```python
from build123d import *

# Parameters (mm, degrees)
SKETCH1_W           = 95.25
SKETCH1_H           = 127
BOSS_EXTRUDE1_DEPTH = 6.35
BOSS_EXTRUDE3_DEPTH = 6.35
SKETCH5_R           = 4.826
CUT_EXTRUDE1_DEPTH  = 7.35
CUT_EXTRUDE2_DEPTH  = 7.35
FILLET9_R           = 5
SKETCH7_R           = 5.453804141
BOSS_EXTRUDE4_DEPTH = 6.35
SKETCH8_W           = 69.85
SKETCH8_H           = 101.6
CUT_EXTRUDE3_DEPTH  = 3.175
SKETCH9_W           = 57.15
SKETCH9_H           = 88.9
CUT_EXTRUDE4_DEPTH  = 4.175
SKETCH11_R          = 1.5875
CUT_EXTRUDE6_DEPTH  = 4.175
CUT_EXTRUDE7_DEPTH  = 3.175
FILLET10_R          = 5
FILLET11_R          = 5
FILLET12_R          = 7.62
SKETCH13_R          = 2.2812375
CUT_EXTRUDE8_DEPTH  = 7.35


with BuildPart() as part:
    # Sketch1 → Boss-Extrude1 (new body)
    with BuildSketch(Plane(origin=(0, 0, 0), x_dir=(1, 0, 0), z_dir=(0, 1, 0))):
        Rectangle(SKETCH1_W, SKETCH1_H)
    extrude(amount=BOSS_EXTRUDE1_DEPTH)

    # Sketch4 → Boss-Extrude3 (add)
    with BuildSketch(Plane(origin=(0, 6.35, 0), x_dir=(1, 0, 0), z_dir=(0, 1, 0))):
        with BuildLine():
            Line((-47.625, 63.5), (-171.916018217, 24.219268021))
            ThreePointArc((-171.916018217, 24.219268021), (-189.6618, 0), (-171.916018217, -24.219268021))
            Line((-171.916018217, -24.219268021), (-47.625, -63.5))
            Line((-47.625, -63.5), (-47.625, 63.5))
        make_face()
    extrude(amount=-BOSS_EXTRUDE3_DEPTH)

    # Sketch5 → Cut-Extrude1 (cut, through all)
    with BuildSketch(Plane(origin=(0, 6.35, 0), x_dir=(1, 0, 0), z_dir=(0, 1, 0))):
        with Locations((-164.2618, 0)):
            Circle(SKETCH5_R)
        with Locations((-8.6868, 0)):
            Circle(SKETCH5_R)
    extrude(amount=-CUT_EXTRUDE1_DEPTH, mode=Mode.SUBTRACT)

    # Sketch6 → Cut-Extrude2 (cut, through all)
    with BuildSketch(Plane(origin=(0, 6.35, 0), x_dir=(1, 0, 0), z_dir=(0, 1, 0))):
        Polygon((-45.72, 50.782905742), (-157.9118, 6.35), (-45.72, 6.35), align=None)
        Polygon((-45.72, -6.35), (-45.72, -50.782905742), (-157.9118, -6.35), align=None)
    extrude(amount=-CUT_EXTRUDE2_DEPTH, mode=Mode.SUBTRACT)

    # Fillet9
    fillet9_edges = [part.edges().sort_by_distance(p)[0] for p in [
        (-45.72, 3.175, -50.782905742),
        (-45.72, 3.175, -6.35),
        (-157.9118, 3.175, -6.35),
        (-157.9118, 3.175, 6.35),
        (-45.72, 3.175, 6.35),
        (-45.72, 3.175, 50.782905742),
    ]]
    fillet(fillet9_edges, radius=FILLET9_R)

    # Sketch7 → Boss-Extrude4 (add)
    with BuildSketch(Plane(origin=(0, 6.35, 0), x_dir=(1, 0, 0), z_dir=(0, 1, 0))):
        with Locations((-8.6868, 0)):
            Circle(SKETCH7_R)
    extrude(amount=-BOSS_EXTRUDE4_DEPTH)

    # Sketch8 → Cut-Extrude3 (cut)
    with BuildSketch(Plane(origin=(0, 6.35, 0), x_dir=(1, 0, 0), z_dir=(0, 1, 0))):
        Rectangle(SKETCH8_W, SKETCH8_H)
    extrude(amount=-CUT_EXTRUDE3_DEPTH, mode=Mode.SUBTRACT)

    # Sketch9 → Cut-Extrude4 (cut, through all)
    with BuildSketch(Plane(origin=(0, 3.175, 0), x_dir=(1, 0, 0), z_dir=(0, 1, 0))):
        Rectangle(SKETCH9_W, SKETCH9_H)
    extrude(amount=-CUT_EXTRUDE4_DEPTH, mode=Mode.SUBTRACT)

    # Sketch11 → Cut-Extrude6 (cut, through all)
    with BuildSketch(Plane(origin=(0, 3.175, 0), x_dir=(1, 0, 0), z_dir=(0, 1, 0))):
        with Locations((-31.75, 0)):
            Circle(SKETCH11_R)
        with Locations((31.75, 0)):
            Circle(SKETCH11_R)
        with Locations((0, 47.625)):
            Circle(SKETCH11_R)
        with Locations((0, -47.625)):
            Circle(SKETCH11_R)
    extrude(amount=-CUT_EXTRUDE6_DEPTH, mode=Mode.SUBTRACT)

    # Sketch12 → Cut-Extrude7 (cut)
    with BuildSketch(Plane(origin=(0, 6.35, 0), x_dir=(1, 0, 0), z_dir=(0, 1, 0))):
        with BuildLine():
            Line((34.925, 7.112), (34.925, -7.112))
            ThreePointArc((34.925, -7.112), (42.037, 0), (34.925, 7.112))
        make_face()
    extrude(amount=-CUT_EXTRUDE7_DEPTH, mode=Mode.SUBTRACT)

    # Fillet10
    fillet10_edges = [part.edges().sort_by_distance(p)[0] for p in [
        (-34.925, 4.7625, -50.8),
        (34.925, 4.7625, -50.8),
        (34.925, 4.7625, 50.8),
        (-34.925, 4.7625, 50.8),
    ]]
    fillet(fillet10_edges, radius=FILLET10_R)

    # Fillet11
    fillet11_edges = [part.edges().sort_by_distance(p)[0] for p in [
        (-28.575, 1.5875, 44.45),
        (-28.575, 1.5875, -44.45),
        (28.575, 1.5875, -44.45),
        (28.575, 1.5875, 44.45),
    ]]
    fillet(fillet11_edges, radius=FILLET11_R)

    # Fillet12
    fillet12_edges = [part.edges().sort_by_distance(p)[0] for p in [
        (47.625, 3.175, 63.5),
        (47.625, 3.175, -63.5),
    ]]
    fillet(fillet12_edges, radius=FILLET12_R)

    # Sketch13 → Cut-Extrude8 (cut, through all)
    with BuildSketch(Plane(origin=(0, 6.35, 0), x_dir=(1, 0, 0), z_dir=(0, 1, 0))):
        with Locations((-43.777254611, 53.125383493)):
            Circle(SKETCH13_R)
        with Locations((-43.777254611, -53.125383493)):
            Circle(SKETCH13_R)
        with Locations((40.602254611, -53.125383493)):
            Circle(SKETCH13_R)
        with Locations((40.602254611, 53.125383493)):
            Circle(SKETCH13_R)
    extrude(amount=-CUT_EXTRUDE8_DEPTH, mode=Mode.SUBTRACT)


solid = part.part
```
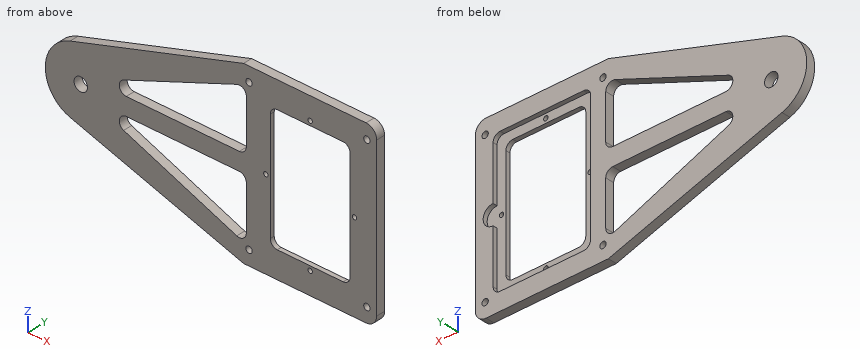
CAD build for the part. Positions are in the model's coordinates, mm. Coordinates: 2 decimals unless noted, no trailing zeros. Order: outer loops, then holes, each group sorted by start corner. A loop starts at its lowest first (then second) coordinate and runs counter-clockwise, first axis right, second up.
(1) Drill centre lines: L1, parallel to Z at x = 0, y = 1.6; L2, parallel to X at y = 1.45, z = 0 (1 decimal); L3, parallel to X at y = 5.5, z = 10 (3 decimals). Where is each one in solid material? Low to high.
Solution:
L1: z = -63.5 to -49.21, -46.04 to -44.45, 44.45 to 46.04, 49.21 to 63.5
L2: x = -189.7 to -169.1, -159.4 to -33.3, -30.2 to -28.6, 28.6 to 30.2, 33.3 to 47.6
L3: x = -187.61 to -136.522, -45.906 to -34.925, 34.925 to 47.625
(2) Saw through at A-A, the plane x = 11.5. Write the cut outline in (y, z) (3 decimals), and give its area (3 significant figures).
Solution:
outline: (0, -63.5) - (6.35, -63.5) - (6.35, -50.8) - (3.175, -50.8) - (3.175, -44.45) - (0, -44.45) - close; (0, 44.45) - (3.175, 44.45) - (3.175, 50.8) - (6.35, 50.8) - (6.35, 63.5) - (0, 63.5) - close
area: 202 mm2
(3) Pin check, flat tips, straight feed: pin 1 Ø5 at (x, z) = (11, -47) entering from +Y (3 decimals); pin 2 Ø1.6 at (y, z) = (4, 19) entering from -X; pin 3 Ø3 at (x, y) = (-140, 4.5) entering from +Z. Stop position of each tip, or through.
Solution:
pin 1: stops at y = 3.175
pin 2: stops at x = -181.98
pin 3: stops at z = 34.78
(4) Saw through at B-B, the plane x = -63.5. Write the cut outline in (y, z).
Solution:
outline: (0, -58.48) - (6.35, -58.48) - (6.35, -43.74) - (0, -43.74) - close; (0, -6.35) - (6.35, -6.35) - (6.35, 6.35) - (0, 6.35) - close; (0, 43.74) - (6.35, 43.74) - (6.35, 58.48) - (0, 58.48) - close
